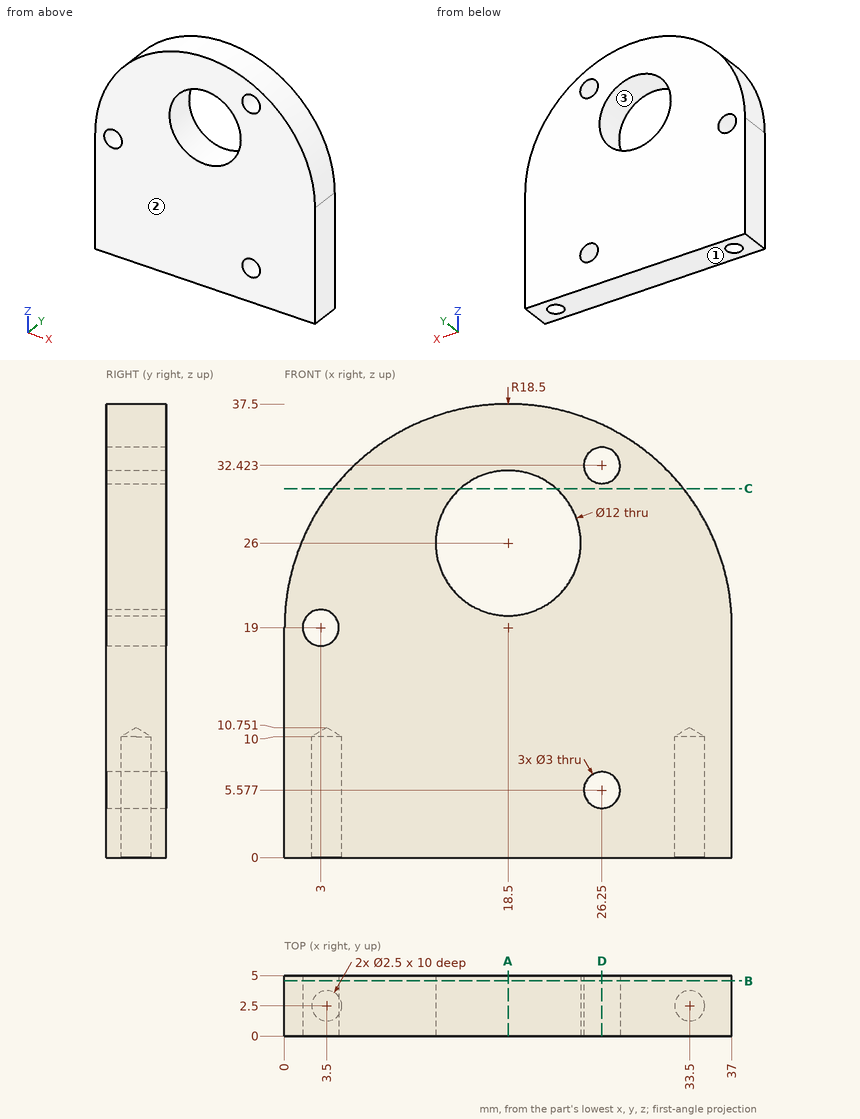
Answer from the drawing. Dimensions are ordinates in mm from the lowest x, y and z of the part. Give positions to 0.01 mm unless a question says otherwise; leave off trailing zeros. Loops run counter-clockwise (first coordinate to the right, second up) from the corner with the lowest first, then second, coordinate; pieces in that order, holes last. Notation, with made-up numbers: (63.25, -15.5) - (98.25, -15.5) arc R30 ccw to (98.25, 9.5) - close; hole circle Ø5 at (-15, 57.25). An arc over 180 degrees is marked (long way). Answer as CSV lines item,"result". Start each with the question number.
Item 1: A cutting plane is placed at D-D on x = 26.25. Determine the outline of the cut face in (y, z), then the cut area to 3 significant figures.
Item 2: Find the intervals of material crossed by line 1 (X direction, y = 2.5, z = 5.5); line 2 (X direction, y = 2.5, z = 4.75); line 3 (X direction, y = 2.65, z = 19), in increasing order. Write a range as from..to.
Item 3: The mould has two halves that part along Z. Classify the marked faces 1, 2 and 3: +Z half, -Z half, draft (parallel to the pull), parting line (faces both ways), or undercut.
Item 4: A cutting plane is placed at B-B on y = 4.55. Determine the outline of the cut face in (x, z).
Item 5: A cutting plane is placed at C-C on z = 30.5. Determine the outline of the cut face in (x, y), then the cut area to 3 significant figures.
Item 6: A cutting plane is placed at A-A on x = 18.5. Determine the outline of the cut face in (y, z).
Item 7: Each of these flat-tipped pins is pushed along its axis until it touches: pin 1 (2 mm diameter, centred on x = 33.5, y = 2.5, fed in from +Z) (1 decimal); pin 2 (1 mm diameter, centred on x = 23.5, y = 3.5, fed in from +Z) (1 decimal). Where does it stop, or does it pass through?
Found:
1,outline,"(0, 0) - (5, 0) - (5, 4.08) - (0, 4.08) - close; (0, 7.08) - (5, 7.08) - (5, 30.92) - (0, 30.92) - close; (0, 33.92) - (5, 33.92) - (5, 35.8) - (0, 35.8) - close"
1,area,"149 mm^2"
2,line 1,"x = 0..2.25, 4.75..24.75, 27.75..32.25, 34.75..37"
2,line 2,"x = 0..2.25, 4.75..25, 27.5..32.25, 34.75..37"
2,line 3,"x = 0..1.5, 4.5..37"
3,face 1,"-Z half"
3,face 2,"draft"
3,face 3,"undercut"
4,outline,"(0, 0) - (37, 0) - (37, 19) arc R18.5 ccw to (0, 19) - close; hole circle Ø3 at (3, 19); hole circle Ø12 at (18.5, 26); hole circle Ø3 at (26.25, 5.58); hole circle Ø3 at (26.25, 32.42)"
5,outline,"(4.01, 0) - (14.53, 0) - (14.53, 5) - (4.01, 5) - close; (22.47, 0) - (32.99, 0) - (32.99, 5) - (22.47, 5) - close"
5,area,"105 mm^2"
6,outline,"(0, 0) - (5, 0) - (5, 20) - (0, 20) - close; (0, 32) - (5, 32) - (5, 37.5) - (0, 37.5) - close"
7,pin 1,"stops at z = 31.1"
7,pin 2,"stops at z = 36.9"
